Geometry check sheet. Reference: drawing and pictorial views, mm from the part's lowest x, y, z. A direction names the side the tool comes from. Give positions to 0.01 mm unless a question says otherwise; leave off trailing zeros. Write each loop counter-clockwise with the first axis right and the second up, starting at its lowest first coordinate (ties: lowest second). Pieces come first, ordered by that corner, then holes. Notation, with made-up numbers: M 41.25,65.5 L 58.25,65.5 A32 cw 58.25,96.5 Z; hole C 7.5,-18.75 d1. An arc over 180 degrees is marked long. Write item = value, one per line. Start each with the question number.
1) Mould release check, pull along Y, two halves, no side actions. Record for the marked faces 4, 5 and 6: released by +Y, released by -Y, zero draft, split by the parting line, or undercut.
2) Cross-section at B-B, the plane z = 10. Record the cut outline in (x, y).
3) Go/stop test with flat-tipped pins: pin 1 (3 mm diameter, centred on x = 46, z = 34.5, fed in from +Y); pin 2 (6 mm diameter, centred on x = 14, y = 26, fed in from +Z); pin 3 (10 mm diameter, centred on x = 21, y = 18.5, fed in from +Z). Record where each tip stops, or that it passes through.
4) Cross-section at C-C, the plane x = 39. Record the cut outline in (y, z).
5) Cross-section at D-D, the plane y = 10.75. Record the cut outline in (x, z).
6) Cross-section at A-A, the plane x = 52. Record the cut outline in (y, z).
7) Scan lines: line 1 along X through (y, z) = (3.05, 10); line 2 along Y through (x, z) = (13, 11); line 3 along Y through (x, z) = (25, 22.5). Record each from-to range of solid material in increasing order. Write a range as [from, to].
8) Access from +Z, -Z, +X, -X, +Y, -Y to the whole of each face (thin tool, end or side, straight path). Record for the marked faces 1, 2 and 3.
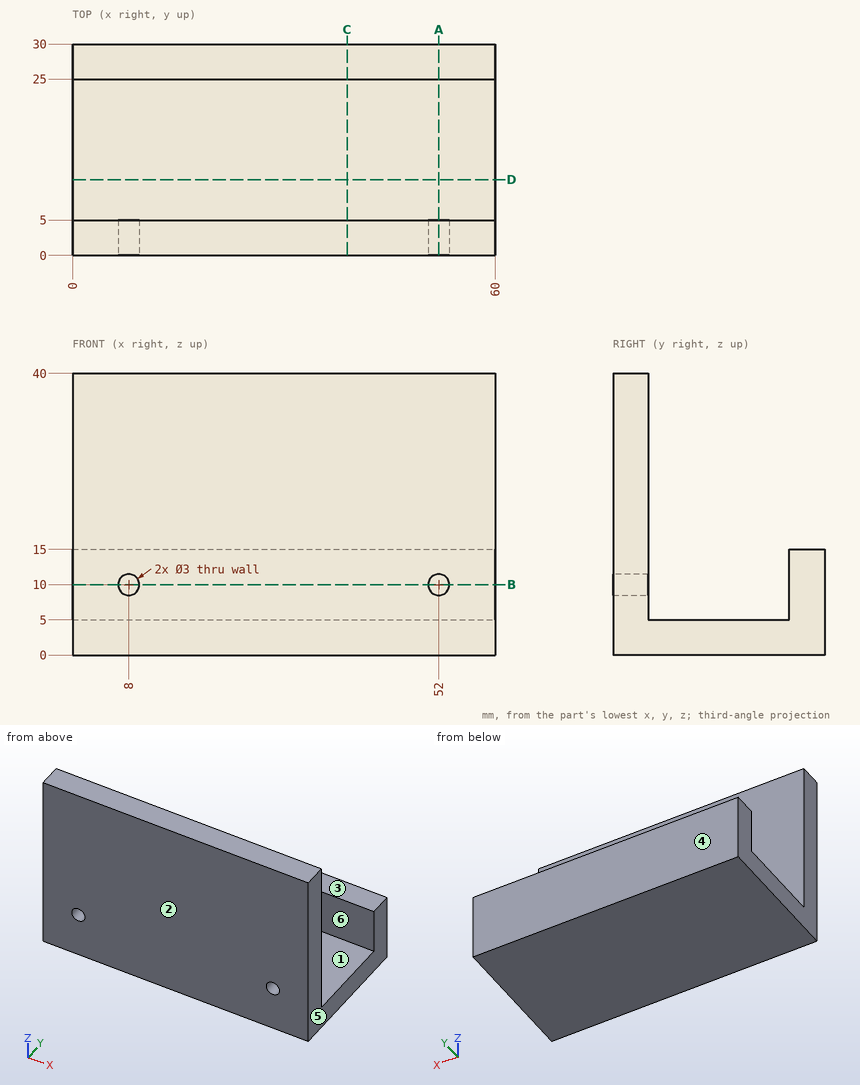
Reply:
q1.face_4 = released by +Y
q1.face_5 = zero draft
q1.face_6 = undercut
q2.outline = M 0,0 L 6.5,0 L 6.5,5 L 0,5 Z; M 0,25 L 60,25 L 60,30 L 0,30 Z; M 9.5,0 L 50.5,0 L 50.5,5 L 9.5,5 Z; M 53.5,0 L 60,0 L 60,5 L 53.5,5 Z
q3.pin_1 = 5
q3.pin_2 = 15
q3.pin_3 = 5
q4.outline = M 0,0 L 30,0 L 30,15 L 25,15 L 25,5 L 5,5 L 5,40 L 0,40 Z
q5.outline = M 0,0 L 60,0 L 60,5 L 0,5 Z
q6.outline = M 0,0 L 30,0 L 30,15 L 25,15 L 25,5 L 5,5 L 5,8.5 L 0,8.5 Z; M 0,11.5 L 5,11.5 L 5,40 L 0,40 Z
q7.line_1 = [0, 6.5], [9.5, 50.5], [53.5, 60]
q7.line_2 = [0, 5], [25, 30]
q7.line_3 = [0, 5]
q8.face_1 = +Z, +X, -X
q8.face_2 = +Z, -Z, +X, -X, -Y
q8.face_3 = +Z, +X, -X, +Y
